from build123d import *

# Parameters (mm, degrees)
SKETCH1_W           = 8
SKETCH1_H           = 10
BOSS_EXTRUDE1_DEPTH = 595
SKETCH2_R           = 1.75
CUT_EXTRUDE1_DEPTH  = 596.097471008
LPATTERN1_COUNT     = 24
LPATTERN1_PITCH     = 25


with BuildPart() as part:
    # Sketch1 → Boss-Extrude1 (new body)
    with BuildSketch(Plane.XY):
        Rectangle(SKETCH1_W, SKETCH1_H)
    extrude(amount=BOSS_EXTRUDE1_DEPTH)

    # Sketch2 → Cut-Extrude1 (cut, through all)
    with BuildSketch(Plane(origin=(0, 5, 0), x_dir=(1, 0, 0), z_dir=(0, 1, 0))):
        with Locations(Location((0, -10, 0), (0, 0, 270))):
            Circle(SKETCH2_R)
    cut_extrude1 = extrude(amount=-CUT_EXTRUDE1_DEPTH, mode=Mode.SUBTRACT)

    # LPattern1: Cut-Extrude1 ×24
    with Locations(*[(0, 0, i * LPATTERN1_PITCH) for i in range(1, LPATTERN1_COUNT)]):
        add(cut_extrude1, mode=Mode.SUBTRACT)


solid = part.part
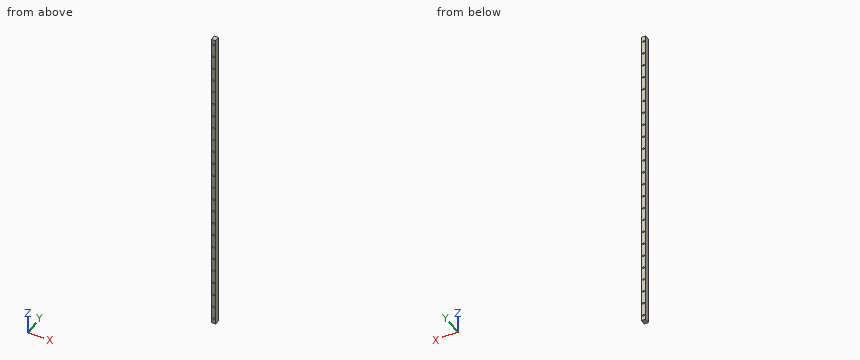
Design review of the part built by this model. Coordinates are the model's own, in mm. Round coordinates to 2 decimals unless told otherwise and drop trailing zeros.
1) Consider section A-A (y = 1.25). Count the separate pieces of the cut face and the enclosed holes in it, plus the area to 3 significant figures.
The answers:
separate pieces: 1
enclosed holes: 24
area: 4,530 mm2
2) For L1, parallel to X at y = -2.5, z = 560; L2, parallel to X at y = 2.5, z = 83.5, list the stretches that pass through material, from the lowest coordinate up.
The answers:
L1: x = -4 to -1.75, 1.75 to 4
L2: x = -4 to -0.9, 0.9 to 4
3) Clearance check with a flat-ended pin moving along its axis: pin 1 Ø2 at (x, z) = (0, 435) entering from +Y. State where the tip first meets the part, or that it passes through.
The answers:
pin 1: passes through
